Part print with two shaded views. Sizes in mm from the minimum x, y, z corner. A direction names the side the tool comes from. Round coordinates to 2 decimals unless told otherwise and drop trailing zeros. Order: outer loops, then holes, each group sorted by start corner. A loop starts at its lowest first (then second) coordinate and runs counter-clockwise, first axis right, second up. Notation, with made-up numbers: (78.25, 28) -> (110.25, 28) arc R25 cw to (110.25, 67) -> close; hole circle Ø5 at (-36.5, 35). An arc over 180 degrees is marked (long way). Put each result on its own line as item: value. Start each with the question number.
Q1. Cut at C-C, the plane y = 25.4. List the corners of the cut face in (x, z).
Q2. Flat gauge pins, fed straight in: P1, Ø10, axis at x = 7.5, y = 21, coming from the +Z side; P2, Ø2, axis at y = 8, z = 13, coming from the +X side; P3, Ø9, axis at x = 38.1, z = 19.05, coming from the -Y side; P4, Ø3, axis at x = 5, z = 9, coming from the +Y side. Where does each tip first touch, or does it go through?
Q3. Probe L1, parallel to X at y = 1, z = 19; L2, parallel to Z at x = 12.7, y = 1.5; L3, parallel to Y at x = 25.4, z = 2.5. List the from-to ranges inside material, lowest first.
Q4. Cut at A-A, the plane z = 19.05. List the corners of the cut face in (x, y), and give its area (3 significant figures).
Q5. 3-axis set-ups, long thin cutter, end or side, ignore diameter. For the marked faces 5 and 6: which of +Z, -Z, +X, -X, +Y, -Y reach the whole face in a straight line?
Q6. Pull direction X, two halves, no side cores. Call the marked faces 1, 2, 3 and 4: released by +X, released by -X, zero draft, split by the parting line, or undercut.
Q7. Cut at B-B, the plane x = 25.4. List the corners of the cut face in (y, z).
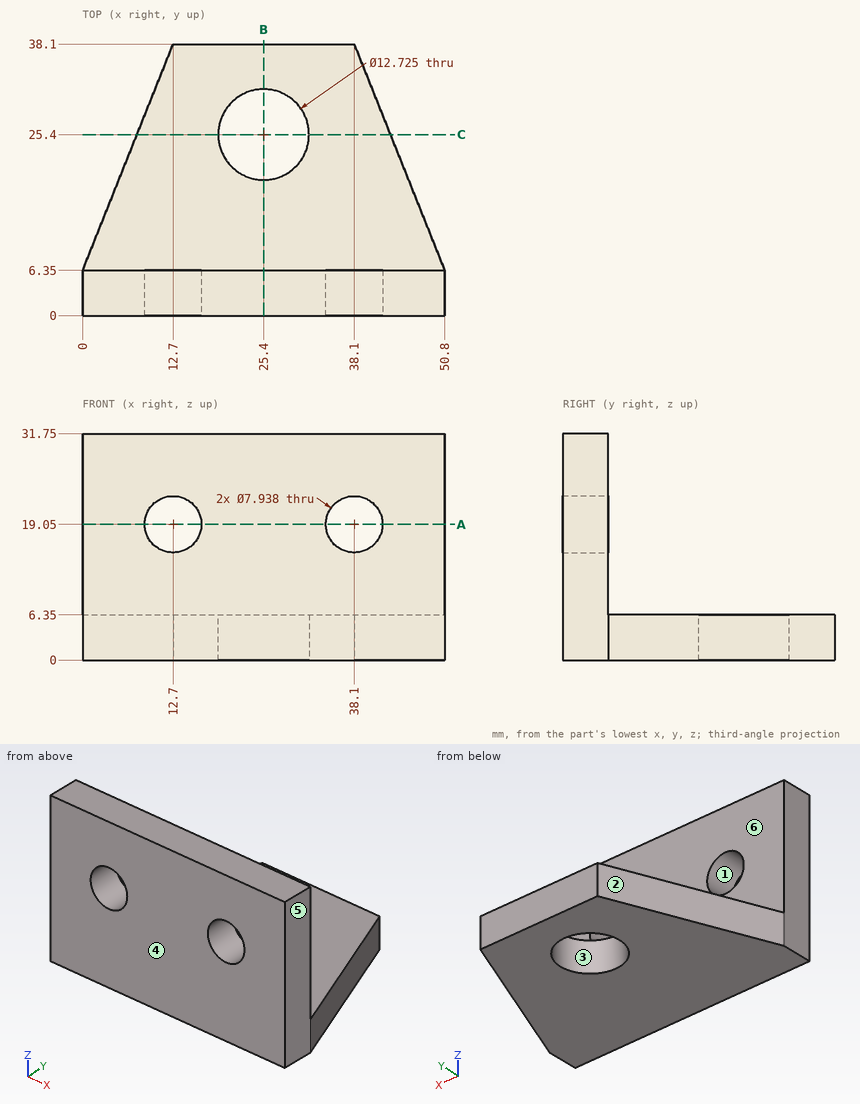
Ans:
1. outline: (7.62, 0) -> (19.04, 0) -> (19.04, 6.35) -> (7.62, 6.35) -> close; (31.76, 0) -> (43.18, 0) -> (43.18, 6.35) -> (31.76, 6.35) -> close
2. P1: stops at z = 6.35
2. P2: passes through
2. P3: stops at y = 0
2. P4: stops at y = 6.35
3. L1: x = 0 to 8.73, 16.67 to 34.13, 42.07 to 50.8
3. L2: z = 0 to 15.08, 23.02 to 31.75
3. L3: y = 0 to 19.04, 31.76 to 38.1
4. outline: (0, 0) -> (8.73, 0) -> (8.73, 6.35) -> (0, 6.35) -> close; (16.67, 0) -> (34.13, 0) -> (34.13, 6.35) -> (16.67, 6.35) -> close; (42.07, 0) -> (50.8, 0) -> (50.8, 6.35) -> (42.07, 6.35) -> close
4. area: 222 mm^2
5. face 5: +Z, -Z, +X, +Y, -Y
5. face 6: +Z, +X, -X, +Y
6. face 1: undercut
6. face 2: released by -X
6. face 3: undercut
6. face 4: zero draft
7. outline: (0, 0) -> (19.04, 0) -> (19.04, 6.35) -> (6.35, 6.35) -> (6.35, 31.75) -> (0, 31.75) -> close; (31.76, 0) -> (38.1, 0) -> (38.1, 6.35) -> (31.76, 6.35) -> close
